The drawing under review shows one solid part. Ordinate dimensions are in mm from its lowest x, y, z. A direction names the side the tool comes from. Give positions to 0.01 mm unless a question says otherwise; leave off trailing zeros. Order: outer loops, then holes, each group sorted by start corner. A loop starts at its lowest first (then second) coordinate and runs counter-clockwise, first axis right, second up. Notation, with made-up numbers: (52.5, 39) -> (80.5, 39) arc R21 cw to (80.5, 44) -> close; hole circle Ø4 at (17, 79). An arc over 180 degrees is marked (long way). One line per item, written item: value.
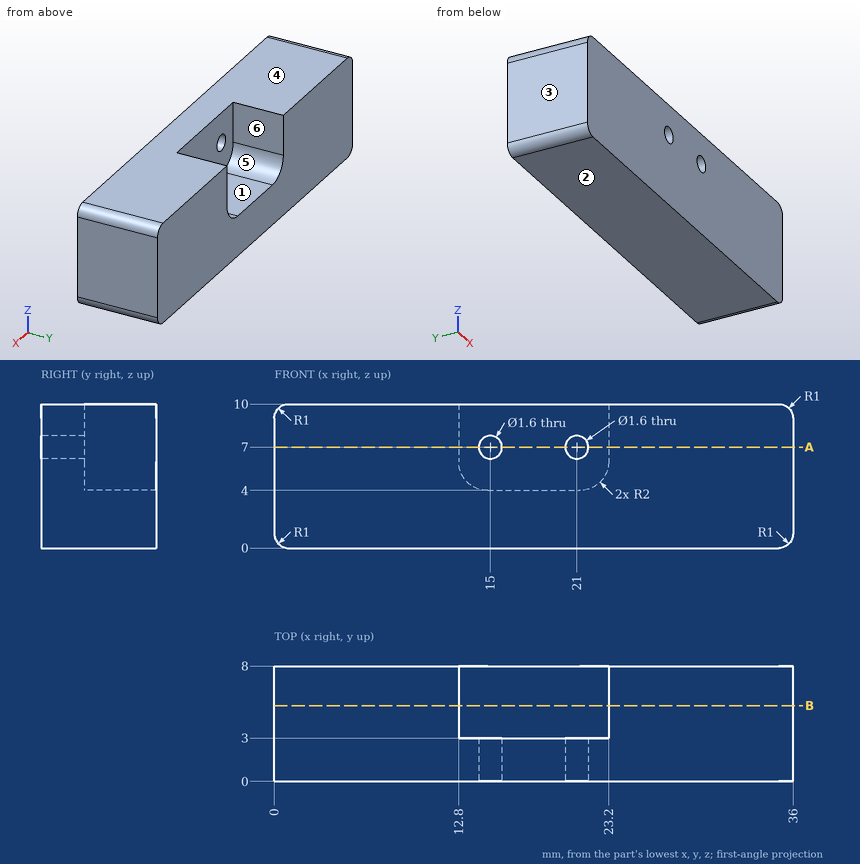
Item 1: To check wall thickness, follow line 1 along X through (y, z) = (2.2, 7); line 2 along X through (y, z) = (6.5, 8.75); line 3 along Y through (x, z) = (13, 9.5). State the ranges of each line that lie inside material, in increasing order. Write a range as from..to.
Returned:
line 1: 0..14.2, 15.8..20.2, 21.8..36
line 2: 0..12.8, 23.2..36
line 3: 0..3
Item 2: Add section A-A on z = 7. Give the boundary of the cut face in (x, y).
Returned:
outline: (0, 0) -> (14.2, 0) -> (14.2, 3) -> (12.8, 3) -> (12.8, 8) -> (0, 8) -> close; (15.8, 0) -> (20.2, 0) -> (20.2, 3) -> (15.8, 3) -> close; (21.8, 0) -> (36, 0) -> (36, 8) -> (23.2, 8) -> (23.2, 3) -> (21.8, 3) -> close
Item 3: Clearance check with flat-ended pins moving along their axes: P1, Ø3, axis at x = 19, z = 6.5, coming from the +Y side; P2, Ø1.3, axis at x = 15, z = 7, coming from the +Y side. State where each tip first meets the part, or that it passes through.
Returned:
P1: y = 3
P2: through
Item 4: Add section B-B on y = 5.25. Give the boundary of the cut face in (x, z).
Returned:
outline: (0, 1) arc R1 ccw to (1, 0) -> (35, 0) arc R1 ccw to (36, 1) -> (36, 9) arc R1 ccw to (35, 10) -> (23.2, 10) -> (23.2, 6) arc R2 cw to (21.2, 4) -> (14.8, 4) arc R2 cw to (12.8, 6) -> (12.8, 10) -> (1, 10) arc R1 ccw to (0, 9) -> close
Item 5: Machinability: for the marked faces 1 and 2, which of the approach directions +Z, -Z, +X, -X, +Y, -Y give a long, thin tool a straight path to every point of the face, cutting with its end or side? Answer none if there is none.
Returned:
face 1: +Z, +Y
face 2: -Z, +X, -X, +Y, -Y
Item 6: Draft analysis for pull direction X (two halves, no side actions). For the marked faces 3, 4, 5 and 6, state which applies: pulls with the +X half, pulls with the -X half, needs draft (parallel to the pull), parting line crosses it, or undercut.
Returned:
face 3: pulls with the -X half
face 4: needs draft
face 5: undercut
face 6: undercut
